Read the model definition and answer for the solid it produces. Units are mm, in the model's axes. A direction names the side the tool comes from. Round coordinates to 2 decimals unless told otherwise and drop trailing zeros. Loops run counter-clockwise (first coordinate to the right, second up) from the corner with the lowest first, then second, coordinate; pieces in that order, holes last. Notation, with made-up numbers: M 20,88.5 L 37,88.5 A23 ccw 37,106.5 Z; hole C 29.5,59 d5. An arc over 180 degrees is marked long. Write each question's results on one line, items separated by ' | '.
```python
from build123d import *

# Parameters (mm, degrees)
SKETCH_4_R          = 12.5
EXTRUDE_1_DEPTH     = 4
SKETCH_5_R          = 2.5
CUT_EXTRUDE_1_DEPTH = 3
SKETCH_6_R          = 14
EXTRUDE_2_DEPTH     = 1
SKETCH_7_R          = 1
CUT_EXTRUDE_2_DEPTH = 2
SKETCH_11_R         = 1
CUT_EXTRUDE_5_DEPTH = 23.797075308
SKETCH_13_R         = 4
SKETCH_13_R_2       = 2.977192395
SKETCH_13_R_3       = 2.5
CUT_EXTRUDE_6_DEPTH = 1.5
CUT_EXTRUDE_7_DEPTH = 2
CHAMFER_2_SIZE      = 0.5
CHAMFER_1_SIZE      = 2
SKETCH_16_R         = 3.5
CUT_EXTRUDE_8_DEPTH = 0.5


with BuildPart() as part:
    # 草图4 → 凸台-拉伸1 (new body)
    with BuildSketch(Plane.XY.offset(20.116672725)):
        with Locations((0.173765051, -3.140916746)):
            Circle(SKETCH_4_R)
    extrude(amount=-EXTRUDE_1_DEPTH)

    # 草图5 → 切除-拉伸1 (cut)
    with BuildSketch(Plane(origin=(0, 0, 16.116672725), x_dir=(-1, 0, 0), z_dir=(0, 0, -1))):
        with Locations((-0.173765051, -3.140916746)):
            Circle(SKETCH_5_R)
    extrude(amount=-CUT_EXTRUDE_1_DEPTH, mode=Mode.SUBTRACT)

    # 草图6 → 凸台-拉伸2 (add)
    with BuildSketch(Plane.XY.offset(20.116672725)):
        with Locations((0.173765051, -3.140916746)):
            Circle(SKETCH_6_R)
    extrude(amount=EXTRUDE_2_DEPTH)

    # 草图7 → 切除-拉伸2 (cut)
    with BuildSketch(Plane(origin=(0, 0, 16.116672725), x_dir=(-1, 0, 0), z_dir=(0, 0, -1))):
        with Locations((-0.173765051, 5.359083254)):
            Circle(SKETCH_7_R)
        with Locations((7.187450882, 1.109083254)):
            Circle(SKETCH_7_R)
        with Locations((7.187450882, -7.390916746)):
            Circle(SKETCH_7_R)
        with Locations((-0.173765051, -11.640916746)):
            Circle(SKETCH_7_R)
        with Locations((-7.534980983, -7.390916746)):
            Circle(SKETCH_7_R)
        with Locations((-7.534980983, 1.109083254)):
            Circle(SKETCH_7_R)
    extrude(amount=-CUT_EXTRUDE_2_DEPTH, mode=Mode.SUBTRACT)

    # 草图11 → 切除-拉伸5 (cut, through all)
    with BuildSketch(Plane.XY.offset(21.116672725)):
        with Locations(Location((0.173765051, -11.640916746, 0), (0, 0, 180))):
            Circle(SKETCH_11_R)
        with Locations(Location((-7.187450882, 1.109083254, 0), (0, 0, 180))):
            Circle(SKETCH_11_R)
        with Locations(Location((7.534980983, 1.109083254, 0), (0, 0, 180))):
            Circle(SKETCH_11_R)
    extrude(amount=-CUT_EXTRUDE_5_DEPTH, mode=Mode.SUBTRACT)

    # 草图13 → 切除-拉伸6 (cut)
    # profile 1 of 4: a face of its own
    with BuildSketch(Plane.XY.offset(21.116672725)):
        with Locations((0.173765051, -3.140916746)):
            Circle(SKETCH_13_R)
        with Locations((0.173765051, -3.140916746)):
            Circle(SKETCH_13_R_2, mode=Mode.SUBTRACT)
    # profile 2 of 4: a face of its own
    with BuildSketch(Plane.XY.offset(21.116672725)):
        with Locations((0.173765051, -11.640916746)):
            Circle(SKETCH_13_R_3)
    # profile 3 of 4: a face of its own
    with BuildSketch(Plane.XY.offset(21.116672725)):
        with Locations((-7.187450882, 1.109083254)):
            Circle(SKETCH_13_R_3)
    # profile 4 of 4: a face of its own
    with BuildSketch(Plane.XY.offset(21.116672725)):
        with Locations((7.534980983, 1.109083254)):
            Circle(SKETCH_13_R_3)
    extrude(amount=-CUT_EXTRUDE_6_DEPTH, mode=Mode.SUBTRACT)

    # 草图15 → 切除-拉伸7 (cut)
    with BuildSketch(Plane.XY.offset(21.116672725)):
        with BuildLine():
            Line((-5.622832862, -11.565446955), (-3.870986227, -9.176206785))
            ThreePointArc((-3.870986227, -9.176206785), (-3.779061338, -8.81107053), (-3.967934532, -8.485338144))
            ThreePointArc((-3.967934532, -8.485338144), (-5.681778189, -6.521616212), (-6.52548944, -4.0555231))
            ThreePointArc((-6.52548944, -4.0555231), (-6.713145364, -3.729087923), (-7.075325081, -3.626129085))
            Line((-7.075325081, -3.626129085), (-10.020391082, -3.94865269))
            ThreePointArc((-10.020391082, -3.94865269), (-10.358840265, -4.136415806), (-10.461871079, -4.509494201))
            ThreePointArc((-10.461871079, -4.509494201), (-9.112909279, -8.50258067), (-6.329275857, -11.667359093))
            ThreePointArc((-6.329275857, -11.667359093), (-5.954665083, -11.764670987), (-5.622832862, -11.565446955))
        make_face()
        with BuildLine():
            Line((-4.223793169, 6.091349407), (-3.030573803, 3.379585632))
            ThreePointArc((-3.030573803, 3.379585632), (-2.760318975, 3.117408215), (-2.383789858, 3.118111006))
            ThreePointArc((-2.383789858, 3.118111006), (0.173765051, 3.620482186), (2.731319959, 3.118111006))
            ThreePointArc((2.731319959, 3.118111006), (3.107849076, 3.117408215), (3.378103905, 3.379585632))
            Line((3.378103905, 3.379585632), (4.57132327, 6.091349407))
            ThreePointArc((4.57132327, 6.091349407), (4.577940233, 6.478336555), (4.306360273, 6.754103056))
            ThreePointArc((4.306360273, 6.754103056), (0.173765051, 7.582411102), (-3.958830172, 6.754103056))
            ThreePointArc((-3.958830172, 6.754103056), (-4.230410131, 6.478336555), (-4.223793169, 6.091349407))
        make_face()
        with BuildLine():
            Line((10.367921183, -3.94865269), (7.422855183, -3.626129085))
            ThreePointArc((7.422855183, -3.626129085), (7.060675465, -3.729087923), (6.873019541, -4.0555231))
            ThreePointArc((6.873019541, -4.0555231), (6.02930829, -6.521616212), (4.315464633, -8.485338144))
            ThreePointArc((4.315464633, -8.485338144), (4.126591439, -8.81107053), (4.218516329, -9.176206785))
            Line((4.218516329, -9.176206785), (5.970362964, -11.565446955))
            ThreePointArc((5.970362964, -11.565446955), (6.302195184, -11.764670987), (6.676805959, -11.667359093))
            ThreePointArc((6.676805959, -11.667359093), (9.46043938, -8.50258067), (10.809401181, -4.509494201))
            ThreePointArc((10.809401181, -4.509494201), (10.706370366, -4.136415806), (10.367921183, -3.94865269))
        make_face()
    extrude(amount=-CUT_EXTRUDE_7_DEPTH, mode=Mode.SUBTRACT)

    # 倒角2
    chamfer_2_edges = [part.edges().sort_by_distance(p)[0] for p in [
        (-13.826234949, -3.140916746, 21.116672725),
        (-2.760318975, 3.117408215, 21.116672725),
        (0.173765051, 3.620482186, 21.116672725),
        (3.107849076, 3.117408215, 21.116672725),
        (3.974713587, 4.73546752, 21.116672725),
        (4.577940233, 6.478336555, 21.116672725),
        (0.173765051, 7.582411102, 21.116672725),
        (-4.230410131, 6.478336555, 21.116672725),
        (-3.627183486, 4.73546752, 21.116672725),
        (-3.779061338, -8.81107053, 21.116672725),
        (-5.681778189, -6.521616212, 21.116672725),
        (-6.713145364, -3.729087923, 21.116672725),
        (-8.547858082, -3.787390887, 21.116672725),
        (-10.358840265, -4.136415806, 21.116672725),
        (-9.112909279, -8.50258067, 21.116672725),
        (-5.954665083, -11.764670987, 21.116672725),
        (-4.746909545, -10.37082687, 21.116672725),
        (5.034980983, 1.109083254, 21.116672725),
        (-9.687450882, 1.109083254, 21.116672725),
        (-2.326234949, -11.640916746, 21.116672725),
        (-3.826234949, -3.140916746, 21.116672725),
        (-2.803427344, -3.140916746, 21.116672725),
        (7.060675465, -3.729087923, 21.116672725),
        (6.02930829, -6.521616212, 21.116672725),
        (4.126591439, -8.81107053, 21.116672725),
        (5.094439646, -10.37082687, 21.116672725),
        (6.302195184, -11.764670987, 21.116672725),
        (9.46043938, -8.50258067, 21.116672725),
        (10.706370366, -4.136415806, 21.116672725),
        (8.895388183, -3.787390887, 21.116672725),
    ]]
    chamfer(chamfer_2_edges, length=CHAMFER_2_SIZE)

    # Chamfer 1
    chamfer_1_edges = [part.edges().sort_by_distance(p)[0] for p in [
        (-12.326234949, -3.140916746, 16.116672725),
    ]]
    chamfer(chamfer_1_edges, length=CHAMFER_1_SIZE)

    # 草图16 → 切除-拉伸8 (cut)
    with BuildSketch(Plane(origin=(0, 0, 16.116672725), x_dir=(-1, 0, 0), z_dir=(0, 0, -1))):
        with Locations((-0.173765051, -3.140916746)):
            Circle(SKETCH_16_R)
    extrude(amount=-CUT_EXTRUDE_8_DEPTH, mode=Mode.SUBTRACT)


solid = part.part
```
1. Find section A-A, the plane z = 17.75. Give the vertices of the cut face in (x, y).
Completed:
outline: C 0.17,-3.14 d24.27; hole C -7.19,-7.39 d2; hole C -7.19,1.11 d2; hole C 0.17,-3.14 d5; hole C 0.17,-11.64 d2; hole C 0.17,5.36 d2; hole C 7.53,-7.39 d2; hole C 7.53,1.11 d2
2. Which of the six approach directions +Z, -Z, +X, -X, +Y, -Y give full straight-line access (tool end or side, diameter ignored) to faces 3 (the face through (9.431, -8.554, 19.877)), 4 (the face through (-7, -7, 18.117))?
Completed:
face 3: +Z | face 4: -Z
3. Given P1, Ø2, axis at y = -6, z = 19.5, coming from the -X side; P2, Ø1, axis at x = -9, z = 19.5, coming from the +Y side; P3, Ø1.8, axis at x = 0.17, y = 5.36, coming from the -Z side; P4, Ø1.8, axis at x = 0.17, y = -11.64, coming from the -Z side, each flat-ended and moving along its own axis, determine where each tip first touches the part or whether it passes through.
Completed:
P1: stops at x = -13.67 | P2: stops at y = 5.86 | P3: stops at z = 18.12 | P4: passes through
4. Determine the mould class of faces 1 (the face through (0, -8, 16.117)), 2 (the face through (6.048, -6.49, 19.877)) for opening direction X: released by +X, released by -X, zero draft, split by the parting line, or undercut.
Completed:
face 1: zero draft | face 2: undercut
5. Find the intervals of material crossed by L1, parallel to Y at x = 6.75, z = 17.85; L2, parallel to Y at x = -5.5, z = 20.55; L3, parallel to X at y = 1.5, z = 17.9, in increasing order.
Completed:
L1: y = -13.46 to -8.01, -6.77 to 0.49, 1.73 to 7.17 | L2: y = -15.94 to -11.4, -6.82 to -0.74, 2.95 to 9.66 | L3: x = -11.2 to -8.11, -6.27 to 6.61, 8.46 to 11.55
